Geometry check sheet. Reference: the model listing, model coordinates, mm. A direction names the side the tool comes from. Give positions to 0.01 mm unless a question says otherwise; leave off trailing zeros. Write each loop counter-clockwise with the first axis right and the second up, starting at its lowest first coordinate (ties: lowest second). Pieces come first, ordered by that corner, then holes. Notation, with made-up numbers: M 69.5,-37 L 77.5,-37 A29 cw 77.5,-11 Z; hole C 14.25,28 d5. An arc over 180 degrees is marked long. Write each question's results on one line, items separated by ' | '.
```python
from build123d import *

# Parameters (mm, degrees)
SKETCH1_R           = 13.4239
BOSS_EXTRUDE1_DEPTH = 1.8796
BOSS_EXTRUDE2_DEPTH = 1.8796
SKETCH3_R           = 11.4046
CUT_EXTRUDE1_DEPTH  = 0.8128
SKETCH4_R           = 5.8674
BOSS_EXTRUDE3_DEPTH = 0.8128
SKETCH5_R           = 3.9243
CUT_EXTRUDE2_DEPTH  = 2.8796
SKETCH6_R           = 7.7216
BOSS_EXTRUDE4_DEPTH = 1.778
SKETCH7_R           = 6.5532
CUT_EXTRUDE3_DEPTH  = 1.778
BOSS_EXTRUDE5_DEPTH = 2.032
SKETCH9_R           = 0.9271
BOSS_EXTRUDE6_DEPTH = 3.683
CIRPATTERN1_COUNT   = 6


with BuildPart() as part:
    # Sketch1 → Boss-Extrude1 (new body)
    with BuildSketch(Plane(origin=(0, 0, 0), x_dir=(1, 0, 0), z_dir=(0, 1, 0))):
        Circle(SKETCH1_R)
    extrude(amount=BOSS_EXTRUDE1_DEPTH)

    # Sketch2 → Boss-Extrude2 (add)
    with BuildSketch(Plane(origin=(0, 1.8796, 0), x_dir=(1, 0, 0), z_dir=(0, 1, 0))):
        with BuildLine():
            Line((-13.892276606, 5.307740723), (-4.699, 0))
            Line((-4.699, 0), (-13.892276606, -5.307740723))
            ThreePointArc((-13.892276606, -5.307740723), (-12.879269997, -7.43585), (-11.542776606, -9.377194096))
            Line((-11.542776606, -9.377194096), (-2.3495, -4.069453372))
            Line((-2.3495, -4.069453372), (-2.3495, -14.684934819))
            ThreePointArc((-2.3495, -14.684934819), (0, -14.8717), (2.3495, -14.684934819))
            Line((2.3495, -14.684934819), (2.3495, -4.069453372))
            Line((2.3495, -4.069453372), (11.542776606, -9.377194096))
            ThreePointArc((11.542776606, -9.377194096), (12.879269997, -7.43585), (13.892276606, -5.307740723))
            Line((13.892276606, -5.307740723), (4.699, 0))
            Line((4.699, 0), (13.892276606, 5.307740723))
            ThreePointArc((13.892276606, 5.307740723), (12.879269997, 7.43585), (11.542776606, 9.377194096))
            Line((11.542776606, 9.377194096), (2.3495, 4.069453372))
            Line((2.3495, 4.069453372), (2.3495, 14.684934819))
            ThreePointArc((2.3495, 14.684934819), (0, 14.8717), (-2.3495, 14.684934819))
            Line((-2.3495, 14.684934819), (-2.3495, 4.069453372))
            Line((-2.3495, 4.069453372), (-11.542776606, 9.377194096))
            ThreePointArc((-11.542776606, 9.377194096), (-12.879269997, 7.43585), (-13.892276606, 5.307740723))
        make_face()
    extrude(amount=-BOSS_EXTRUDE2_DEPTH)

    # Sketch3 → Cut-Extrude1 (cut)
    with BuildSketch(Plane(origin=(0, 1.8796, 0), x_dir=(1, 0, 0), z_dir=(0, 1, 0))):
        Circle(SKETCH3_R)
    extrude(amount=-CUT_EXTRUDE1_DEPTH, mode=Mode.SUBTRACT)

    # Sketch4 → Boss-Extrude3 (add)
    with BuildSketch(Plane(origin=(0, 1.0668, 0), x_dir=(1, 0, 0), z_dir=(0, 1, 0))):
        Circle(SKETCH4_R)
    extrude(amount=BOSS_EXTRUDE3_DEPTH)

    # Sketch5 → Cut-Extrude2 (cut, through all)
    with BuildSketch(Plane(origin=(0, 1.8796, 0), x_dir=(1, 0, 0), z_dir=(0, 1, 0))):
        Circle(SKETCH5_R)
    extrude(amount=-CUT_EXTRUDE2_DEPTH, mode=Mode.SUBTRACT)

    # Sketch6 → Boss-Extrude4 (add)
    with BuildSketch(Plane.XZ):
        Circle(SKETCH6_R)
    extrude(amount=BOSS_EXTRUDE4_DEPTH)

    # Sketch7 → Cut-Extrude3 (cut)
    with BuildSketch(Plane.XZ.offset(1.778)):
        Circle(SKETCH7_R)
    extrude(amount=-CUT_EXTRUDE3_DEPTH, mode=Mode.SUBTRACT)

    # Sketch8 → Boss-Extrude5 (add)
    with BuildSketch(Plane.XZ):
        with BuildLine():
            Line((-2.3495, -13.216691756), (-2.3495, -14.684934819))
            ThreePointArc((-2.3495, -14.684934819), (0, -14.8717), (2.3495, -14.684934819))
            Line((2.3495, -14.684934819), (2.3495, -13.216691756))
            ThreePointArc((2.3495, -13.216691756), (0, -13.4239), (-2.3495, -13.216691756))
        make_face()
        with BuildLine():
            Line((10.271240814, -8.643072564), (11.542776606, -9.377194096))
            ThreePointArc((11.542776606, -9.377194096), (12.879269997, -7.43585), (13.892276606, -5.307740723))
            Line((13.892276606, -5.307740723), (12.620740814, -4.573619192))
            ThreePointArc((12.620740814, -4.573619192), (11.625438418, -6.71195), (10.271240814, -8.643072564))
        make_face()
        with BuildLine():
            Line((12.620740814, 4.573619192), (13.892276606, 5.307740723))
            ThreePointArc((13.892276606, 5.307740723), (12.879269997, 7.43585), (11.542776606, 9.377194096))
            Line((11.542776606, 9.377194096), (10.271240814, 8.643072564))
            ThreePointArc((10.271240814, 8.643072564), (11.625438418, 6.71195), (12.620740814, 4.573619192))
        make_face()
        with BuildLine():
            Line((2.3495, 13.216691756), (2.3495, 14.684934819))
            ThreePointArc((2.3495, 14.684934819), (0, 14.8717), (-2.3495, 14.684934819))
            Line((-2.3495, 14.684934819), (-2.3495, 13.216691756))
            ThreePointArc((-2.3495, 13.216691756), (0, 13.4239), (2.3495, 13.216691756))
        make_face()
        with BuildLine():
            Line((-10.271240814, 8.643072564), (-11.542776606, 9.377194096))
            ThreePointArc((-11.542776606, 9.377194096), (-12.879269997, 7.43585), (-13.892276606, 5.307740723))
            Line((-13.892276606, 5.307740723), (-12.620740814, 4.573619192))
            ThreePointArc((-12.620740814, 4.573619192), (-11.625438418, 6.71195), (-10.271240814, 8.643072564))
        make_face()
        with BuildLine():
            Line((-12.620740814, -4.573619192), (-13.892276606, -5.307740723))
            ThreePointArc((-13.892276606, -5.307740723), (-12.879269997, -7.43585), (-11.542776606, -9.377194096))
            Line((-11.542776606, -9.377194096), (-10.271240814, -8.643072564))
            ThreePointArc((-10.271240814, -8.643072564), (-11.625438418, -6.71195), (-12.620740814, -4.573619192))
        make_face()
    extrude(amount=BOSS_EXTRUDE5_DEPTH)

    # Sketch9 → Boss-Extrude6 (add)
    with BuildSketch(Plane.XZ):
        with Locations((0, 13.1445)):
            Circle(SKETCH9_R)
    boss_extrude6 = extrude(amount=BOSS_EXTRUDE6_DEPTH)

    # CirPattern1: Boss-Extrude6 ×6 about axis
    cirpattern1_axis = Axis((0, 0, 0), (0, 1, 0))
    for i in range(1, CIRPATTERN1_COUNT):
        add(boss_extrude6.rotate(cirpattern1_axis, i * 360 / CIRPATTERN1_COUNT))


solid = part.part
```
Q1. Section check D-D (x = -8.75). Enter the section's corners in (y, z), then the cut area to 3 significant figures.
Answer key:
outline: M 0,-10.18 L 1.88,-10.18 L 1.88,-7.31 L 1.07,-7.31 L 1.07,7.31 L 1.88,7.31 L 1.88,10.18 L 0,10.18 Z | area: 26.4 mm2
Q2. Access from +Z, -Z, +X, -X, +Y, -Y to the whole of each face (thin tool, end or side, straight path). Record for faces 1 (the face through (-0.03, -2.032, 14.24)), 2 (the face through (2.35, 0, -14)), 3 (the face through (-13.424, 0.927, -0.065)), 4 (the face through (-2.472, 1.479, 11.133)), 5 (the face through (-2.35, 0, -14)).
Answer key:
face 1: +Z, -Y | face 2: -Z, +X, +Y, -Y | face 3: -X, +Y, -Y | face 4: +Y | face 5: -Z, -X, +Y, -Y
Q3. Section check A-A (z = 0). Enter the section's corners in (x, y).
Answer key:
outline: M -13.42,0 L -7.72,0 L -7.72,-1.78 L -6.55,-1.78 L -6.55,0 L -3.92,0 L -3.92,1.88 L -5.87,1.88 L -5.87,1.07 L -11.4,1.07 L -11.4,1.88 L -13.42,1.88 Z; M 3.92,0 L 6.55,0 L 6.55,-1.78 L 7.72,-1.78 L 7.72,0 L 13.42,0 L 13.42,1.88 L 11.4,1.88 L 11.4,1.07 L 5.87,1.07 L 5.87,1.88 L 3.92,1.88 Z
Q4. Release check for a two-part mould opening along X. For faces 6 (the face through (-10.734, -1.002, 8.061)), 7 (the face through (11, -3.683, -7)), 8 (the face through (2.35, 0, 14)) record: released by +X, released by -X, zero draft, split by the parting line, or undercut.
Answer key:
face 6: undercut | face 7: zero draft | face 8: released by +X
Q5. Material ranges on probe 1 along Z at (x, y) = (0, 1.3); probe 2 along X at (y, z) = (1.3, 0); probe 3 along Z at (x, y) = (0, -1.2), recorded low to high. Write a range as [from, to].
Answer key:
probe 1: z = [-14.87, -11.4], [-5.87, -3.92], [3.92, 5.87], [11.4, 14.87] | probe 2: x = [-13.42, -11.4], [-5.87, -3.92], [3.92, 5.87], [11.4, 13.42] | probe 3: z = [-14.87, -12.22], [-7.72, -6.55], [6.55, 7.72], [12.22, 14.87]
Q6. Depth check by flat-ended pin: P1, Ø3, axis at x = -7.5, y = -2, coming from the -Z side; P2, Ø1.6, axis at y = -0.5, z = 14.5, coming from the -X side; P3, Ø1, axis at y = -1, z = -5, coming from the -X side; P4, Ø4.5, axis at x = -3.5, z = -1, coming from the -Y side. Enter the tip coordinate at first touch or a pass-through.
Answer key:
P1: stops at z = -4.84 | P2: stops at x = -2.35 | P3: stops at x = -13.89 | P4: stops at y = 0
Q7. Section check B-B (y = -0.5). State how many separate pieces and enclosed holes the cut face has, then the cut area to 3 significant figures.
Answer key:
separate pieces: 7 | enclosed holes: 1 | area: 104 mm2
